```python
from build123d import *

# Parameters (mm, degrees)
SKETCH1_R               = 27
SKETCH1_R_2             = 1.25
SKETCH1_R_3             = 20
BOSS_EXTRUDE1_DEPTH     = 10
SKETCH3_R               = 20
SKETCH3_R_2             = 1.25
BOSS_EXTRUDE2_DEPTH     = 2
BOSS_EXTRUDE3_DEPTH     = 6
CUT_EXTRUDE1_REACH      = 44.996
CUT_EXTRUDE1_END_RADIUS = 27
SKETCH4_W               = 6
SKETCH4_H               = 4
SKETCH6_W               = 25
SKETCH6_H               = 15.32
BOSS_EXTRUDE4_DEPTH     = 2.5
SKETCH7_R               = 1.5
BOSS_EXTRUDE5_DEPTH     = 2.5
FILLET2_R               = 10
FILLET3_R               = 1


with BuildPart() as part:
    # Sketch1 → Boss-Extrude1 (new body)
    with BuildSketch(Plane.XY):
        Circle(SKETCH1_R)
        with Locations((0, 23.5)):
            Circle(SKETCH1_R_2, mode=Mode.SUBTRACT)
        with Locations((23.5, 0)):
            Circle(SKETCH1_R_2, mode=Mode.SUBTRACT)
        with Locations((0, -23.5)):
            Circle(SKETCH1_R_2, mode=Mode.SUBTRACT)
        with Locations((-23.5, 0)):
            Circle(SKETCH1_R_2, mode=Mode.SUBTRACT)
        Circle(SKETCH1_R_3, mode=Mode.SUBTRACT)
    extrude(amount=BOSS_EXTRUDE1_DEPTH)

    # Sketch3 → Boss-Extrude2 (add)
    with BuildSketch(Plane.XY):
        Circle(SKETCH3_R)
        with Locations((-7, 0)):
            Circle(SKETCH3_R_2, mode=Mode.SUBTRACT)
        with Locations((7, 0)):
            Circle(SKETCH3_R_2, mode=Mode.SUBTRACT)
    extrude(amount=BOSS_EXTRUDE2_DEPTH)

    # Sketch5 → Boss-Extrude3 (add)
    with BuildSketch(Plane.XY.offset(10)):
        Polygon((-12.5, 23.932195888), (-4.251935746, 23.932195888), (0, 26.25446737), (4.267780323, 23.932195888), (12.5, 23.932195888), (12.5, 31.932195888), (-12.5, 31.932195888), align=None)
    extrude(amount=-BOSS_EXTRUDE3_DEPTH)

    # Cut-Extrude1: up to this cylinder (the profile starts inside it)
    cut_extrude1_end = Plane(origin=(0, 0, 5.5), z_dir=(0, 0, -1)) * Cylinder(CUT_EXTRUDE1_END_RADIUS, 144.992, mode=Mode.PRIVATE)
    # Sketch4 → Cut-Extrude1 (cut, up to the surface)
    with BuildSketch(Plane(origin=(0, 0, 0), x_dir=(1, 0, 0), z_dir=(0, 1, 0)), mode=Mode.PRIVATE) as cut_extrude1_sk1:
        with Locations((-9, -5.5)):
            Rectangle(SKETCH4_W, SKETCH4_H)
    cut_extrude1_tool1 = extrude(cut_extrude1_sk1.sketch, amount=-CUT_EXTRUDE1_REACH, mode=Mode.PRIVATE) & cut_extrude1_end
    add(cut_extrude1_tool1.solids().sort_by_distance((-9, 0, 5.5))[0], mode=Mode.SUBTRACT)

    # Sketch6 → Boss-Extrude4 (add)
    with BuildSketch(Plane(origin=(0, 31.932195888, 0), x_dir=(1, 0, 0), z_dir=(0, 1, 0))):
        with Locations((0, -2.34)):
            Rectangle(SKETCH6_W, SKETCH6_H)
    boss_extrude4 = extrude(amount=-BOSS_EXTRUDE4_DEPTH)

    # Sketch7 → Boss-Extrude5 (add)
    with BuildSketch(Plane(origin=(0, 31.932195888, 0), x_dir=(1, 0, 0), z_dir=(0, 1, 0))):
        with BuildLine():
            Line((-36.25, -9.68), (-28.75, -9.68))
            Line((-28.75, -9.68), (0, -9.68))
            Line((0, -9.68), (0, 5.32))
            Line((0, 5.32), (-32.25, 5.32))
            ThreePointArc((-32.25, 5.32), (-35.078427125, 4.148427125), (-36.25, 1.32))
            Line((-36.25, 1.32), (-36.25, -2.18))
            Line((-36.25, -2.18), (-36.25, -9.68))
        make_face()
        with Locations(Location((-28.75, -2.18, 0), (0, 0, 270))):
            Circle(SKETCH7_R, mode=Mode.SUBTRACT)
    boss_extrude5 = extrude(amount=-BOSS_EXTRUDE5_DEPTH)

    # Fillet2
    # the kernel refuses this fillet: 10 mm, written as the material it adds along each edge
    with BuildSketch(Plane(origin=(-12.5, 29.432195888, 9.68), x_dir=(-1, 0, 0), z_dir=(0, 1, 0))) as fillet2_piece_1:
        with BuildLine():
            CenterArc((2.509501943, 10), FILLET2_R, 255.466253099, 14.533746901)
            Line((0, 0.32), (-0.050190039, 0.1264))
            ThreePointArc((-0.050190039, 0.1264), (-0.2, 0.16), (-0.2, 0))
            Line((-0.2, 0), (0, -0.2))
            Line((0, -0.2), (2.509501943, -0.2))
            Line((2.509501943, -0.2), (2.509501943, 0))
        make_face()
    extrude(amount=2.5)

    # Mirror1: Boss-Extrude4, Boss-Extrude5 across plane
    add(boss_extrude4.mirror(Plane(origin=(0, 0, 0), x_dir=(0, 0, 1), z_dir=(1, 0, 0))))
    add(boss_extrude5.mirror(Plane(origin=(0, 0, 0), x_dir=(0, 0, 1), z_dir=(1, 0, 0))))

    # Fillet3
    # the kernel refuses this fillet: 1 mm, written as the material it adds along each edge
    with BuildSketch(Plane(origin=(-12.5, 29.432195888, 4), x_dir=(0, -1, 0), z_dir=(0, 0, 1))) as fillet3_piece_1_section:
        with BuildLine():
            CenterArc((FILLET3_R, -FILLET3_R), FILLET3_R, 90, 90)
            Line((0, -FILLET3_R), (0, 0))
            Line((0, 0), (FILLET3_R, 0))
        make_face()
    fillet3_piece_1 = extrude(amount=6, mode=Mode.PRIVATE)
    fillet3_piece_1 = fillet3_piece_1 - Plane(origin=(-15.009501943, 29.204760134, 19.68), x_dir=(-1, 0, 0), z_dir=(0, -1, 0)) * Cylinder(10, 16, mode=Mode.PRIVATE)
    add(fillet3_piece_1)
    with BuildSketch(Plane(origin=(12.5, 29.432195888, 9.68), x_dir=(0, -1, 0), z_dir=(0, 0, -1))) as fillet3_piece_2:
        with BuildLine():
            CenterArc((FILLET3_R, -FILLET3_R), FILLET3_R, 90, 90)
            Line((0, -FILLET3_R), (0, 0))
            Line((0, 0), (FILLET3_R, 0))
        make_face()
    extrude(amount=5.68)
    with BuildSketch(Plane(origin=(12.5, 29.432195888, 4), x_dir=(0, -1, 0), z_dir=(-1, 0, 0))) as fillet3_piece_3:
        with BuildLine():
            CenterArc((FILLET3_R, -FILLET3_R), FILLET3_R, 90, 90)
            Line((0, -FILLET3_R), (0, 0))
            Line((0, 0), (FILLET3_R, 0))
        make_face()
    extrude(amount=25)
    with BuildSketch(Plane(origin=(-12.5, 29.432195888, 1.5), x_dir=(0, -1, 0), z_dir=(0, 0, 1))) as fillet3_piece_4a_section:
        with BuildLine():
            CenterArc((FILLET3_R, -FILLET3_R), FILLET3_R, 90, 90)
            Line((0, -FILLET3_R), (0, 0))
            Line((0, 0), (FILLET3_R, 0))
        make_face()
    fillet3_piece_4a = extrude(amount=8.5, mode=Mode.PRIVATE)
    fillet3_piece_4a = split(fillet3_piece_4a, bisect_by=Plane(origin=(-12.726395114, 29.205800773, 4), z_dir=(0, 0, -1)), keep=Keep.TOP, mode=Mode.PRIVATE)
    with BuildSketch(Plane(origin=(12.5, 29.432195888, 4), x_dir=(0, -1, 0), z_dir=(-1, 0, 0))) as fillet3_piece_4b_section:
        with BuildLine():
            CenterArc((FILLET3_R, -FILLET3_R), FILLET3_R, 90, 90)
            Line((0, -FILLET3_R), (0, 0))
            Line((0, 0), (FILLET3_R, 0))
        make_face()
    fillet3_piece_4b = extrude(amount=27.5, mode=Mode.PRIVATE)
    fillet3_piece_4b = split(fillet3_piece_4b, bisect_by=Plane(origin=(-12.5, 29.205800773, 3.773604886), z_dir=(-1, 0, 0)), keep=Keep.TOP, mode=Mode.PRIVATE)
    fillet3_piece_4 = fillet3_piece_4a & fillet3_piece_4b
    add(fillet3_piece_4)
    with BuildSketch(Plane(origin=(12.5, 29.432195888, 9.68), x_dir=(0, -1, 0), z_dir=(0, 0, -1))) as fillet3_piece_5a_section:
        with BuildLine():
            CenterArc((FILLET3_R, -FILLET3_R), FILLET3_R, 90, 90)
            Line((0, -FILLET3_R), (0, 0))
            Line((0, 0), (FILLET3_R, 0))
        make_face()
    fillet3_piece_5a = extrude(amount=8.18, mode=Mode.PRIVATE)
    fillet3_piece_5a = split(fillet3_piece_5a, bisect_by=Plane(origin=(12.726395114, 29.205800773, 4), z_dir=(0, 0, -1)), keep=Keep.TOP, mode=Mode.PRIVATE)
    with BuildSketch(Plane(origin=(15, 29.432195888, 4), x_dir=(0, -1, 0), z_dir=(-1, 0, 0))) as fillet3_piece_5b_section:
        with BuildLine():
            CenterArc((FILLET3_R, -FILLET3_R), FILLET3_R, 90, 90)
            Line((0, -FILLET3_R), (0, 0))
            Line((0, 0), (FILLET3_R, 0))
        make_face()
    fillet3_piece_5b = extrude(amount=27.5, mode=Mode.PRIVATE)
    fillet3_piece_5b = split(fillet3_piece_5b, bisect_by=Plane(origin=(12.5, 29.205800773, 3.773604886), z_dir=(1, 0, 0)), keep=Keep.TOP, mode=Mode.PRIVATE)
    fillet3_piece_5 = fillet3_piece_5a & fillet3_piece_5b
    add(fillet3_piece_5)


solid = part.part
```
Source: CAD feature listing. Evaluate the final solid. Frame: model axes, mm. A direction names the side the tool comes from. Coordinates: 2 decimals unless noted, no trailing zeros. Order: outer loops, then holes, each group sorted by start corner. A loop starts at its lowest first (then second) coordinate and runs counter-clockwise, first axis right, second up. Notation, with made-up numbers: M 73.25,31.5 L 116.25,31.5 A11 ccw 116.25,47.5 Z; hole C 31.5,86.5 d6. An arc over 180 degrees is marked long. Write each question's results on one line, items separated by ' | '. Start each with the question number.
1) Contact query for flat-ended pins moving along their axis: pin 1 Ø2 at (x, y) = (-7, 0) entering from -Z; pin 2 Ø3 at (x, y) = (0, 23.5) entering from +Z; pin 3 Ø4 at (x, y) = (26, 31) entering from +Z; pin 4 Ø6.5 at (x, y) = (-10, -22.5) entering from -Z. Output: stop coordinate, or through.
2) Section query A-A (y = 0). Return the cut outline in (x, z).
3) Line query: line 1 (Y direction, x = 0, z = 5.25); line 2 (Y direction, x = 0, z = 0.25); line 3 (X direction, y = 31.1, z = 2.18). Output: solid intervals per line, ascending. Write a range as from..to.
4) Access query for faces 5 (the face through (-12.5, 26, 7)), 6 (the face through (-0.2, 27.2, 4)), 7 (the face through (-26, 31, 9.68)). Directions: +Z, -Z, +X, -X, +Y, -Y. A direction counts if a zero-diameter tool reaches every point of the face in a straight line with its end or side. Return the directions, or none.
5) Draft query along Z for faces 1 (the face through (0, 0, 0)), 2 (the face through (-6, -23, 6)), 3 (the face through (-12, -20, 6)), 4 (the face through (-36.25, 31, 4)). Return one class per face: released by +Z, released by -Z, zero draft, split by the parting line, or undercut.
6) Section query B-B (x = 28.75). Return the cut outline in (y, z), plus the area to 3 significant figures.
7) Section query D-D (x = 7). Return the cut outline in (y, z) (3 decimals).
8) Section query C-C (y = -11). Return the cut outline in (x, z), plus the area to 3 significant figures.
Answers:
1) pin 1: passes through | pin 2: stops at z = 10 | pin 3: stops at z = 9.68 | pin 4: stops at z = 0
2) outline: M -27,0 L -24.75,0 L -24.75,10 L -27,10 Z; M -22.25,0 L -8.25,0 L -8.25,2 L -20,2 L -20,10 L -22.25,10 Z; M -5.75,0 L 5.75,0 L 5.75,2 L -5.75,2 Z; M 8.25,0 L 22.25,0 L 22.25,10 L 20,10 L 20,2 L 8.25,2 Z; M 24.75,0 L 27,0 L 27,10 L 24.75,10 Z
3) line 1: y = -27..-24.75, -22.25..-20, 20..22.25, 24.75..31.93 | line 2: y = -27..-24.75, -22.25..22.25, 24.75..27, 29.43..31.93 | line 3: x = -36.25..-30.25, -27.25..27.25, 30.25..36.25
4) face 5: +Z, -Z, -X | face 6: -Z | face 7: +Z, -X, +Y
5) face 1: released by -Z | face 2: undercut | face 3: undercut | face 4: zero draft
6) outline: M 29.43,-5.32 L 31.93,-5.32 L 31.93,0.68 L 29.43,0.68 Z; M 29.43,3.68 L 31.93,3.68 L 31.93,9.68 L 29.43,9.68 Z | area: 30.0 mm^2
7) outline: M -26.077,0 L -1.25,0 L -1.25,2 L -18.735,2 L -18.735,10 L -26.077,10 Z; M 1.25,0 L 26.077,0 L 26.077,4 L 28.432,4 A1 cw 29.432,3 L 29.432,-5.32 L 31.932,-5.32 L 31.932,10 L 18.735,10 L 18.735,2 L 1.25,2 Z
8) outline: M -24.66,0 L 24.66,0 L 24.66,10 L 16.7,10 L 16.7,2 L -16.7,2 L -16.7,10 L -24.66,10 Z | area: 226 mm^2
